Verification items for this drawing (mm, ordinates from the low corner). Give positions to 0.01 mm unless a question says otherwise; leave off trailing zeros. Loops run counter-clockwise (first coordinate to the right, second up) from the corner with the lowest first, then second, coordinate; pieces in that order, holes last. Notation, with made-up numbers: (46, 86) -> (90, 86) arc R18 ccw to (90, 104) -> close; hole circle Ø10 at (-9.5, 26.25). An arc over 180 degrees is marked (long way). Write each question's results on one line, items separated by ' | '. Start each with the question number.
1) Scan lines: line 1 (Y direction, x = 9.5, z = 6); line 2 (Z direction, x = 4.25, y = 20.25); line 3 (Y direction, x = 4.75, z = 1). Record each from-to range of solid material in increasing order. Write a range as from..to.
2) Sectioned sample at B-B on y = 21.75. Record the cut outline in (x, z).
3) Depth check by flat-ended pin: pin 1 (8 mm diameter, centred on x = 17.5, z = 28, fed in from -Y). Enter the tip coordinate at first touch or a pass-through.
4) Sectioned sample at A-A on z = 2. Record the cut outline in (x, y), then the cut area to 3 significant figures.
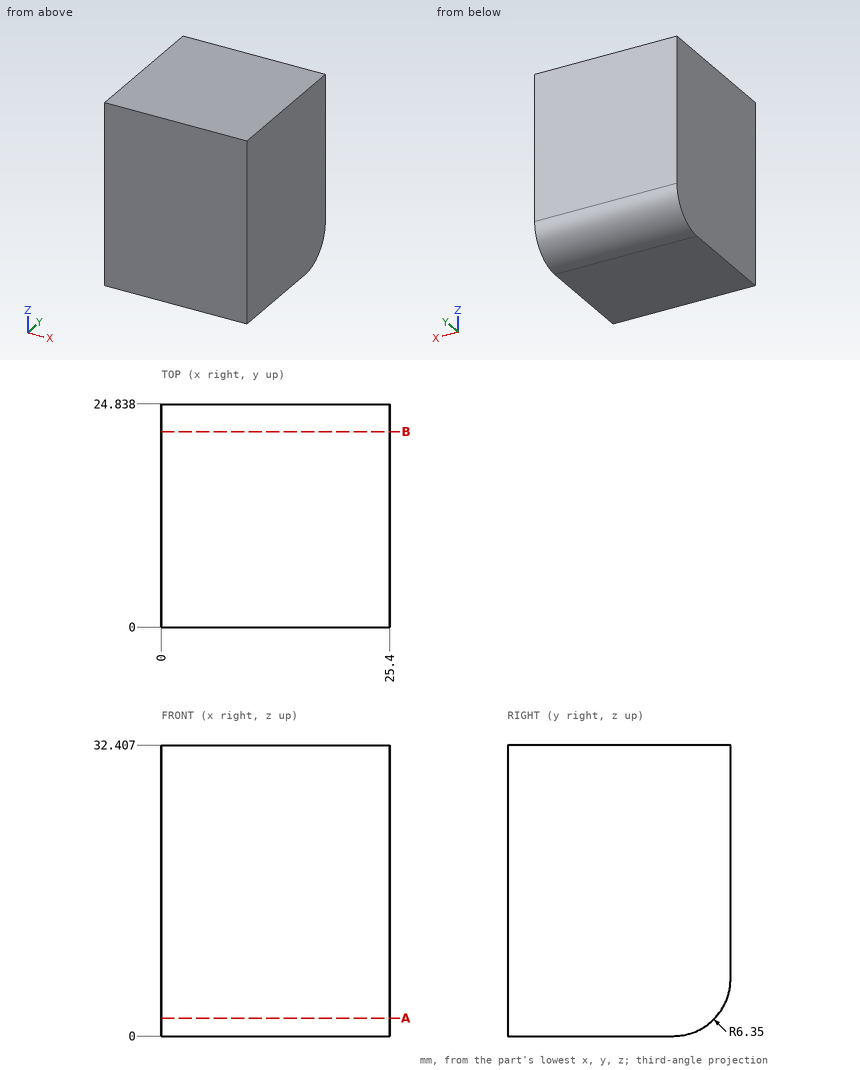
Result:
1) line 1: 0..24.83 | line 2: 0.25..32.41 | line 3: 0..21.91
2) outline: (0, 0.9) -> (25.4, 0.9) -> (25.4, 32.41) -> (0, 32.41) -> close
3) pin 1: y = 0
4) outline: (0, 0) -> (25.4, 0) -> (25.4, 23.11) -> (0, 23.11) -> close | area: 587 mm^2
